```python
from build123d import *

# Parameters (mm, degrees)
SKETCH1_W                       = 123.5
SKETCH1_H                       = 220
BLOCO_DEPTH                     = 20.4
SKETCH2_R                       = 17.5
FURO_35_PASSANTE_DEPTH          = 254.117383836
SKETCH2_4_R                     = 30
SKETCH2_4_R_2                   = 17.5
REBAIXO_60X10_DEPTH             = 10
REBAIXO_M6_PASSANTE_D           = 6.6
REBAIXO_M6_PASSANTE_CBORE_D     = 11
REBAIXO_M6_PASSANTE_CBORE_DEPTH = 6
FURO_M5X0_8_PASSANTE_D          = 4.2


with BuildPart() as part:
    # Sketch1 → Bloco (new body)
    with BuildSketch(Plane(origin=(0, 0, 0), x_dir=(1, 0, 0), z_dir=(0, 1, 0))):
        with Locations((61.75, 110)):
            Rectangle(SKETCH1_W, SKETCH1_H)
    extrude(amount=-BLOCO_DEPTH)

    # Sketch2 → Furo _35 Passante (cut, through all)
    with BuildSketch(Plane(origin=(0, -20.4, 0), x_dir=(-1, 0, 0), z_dir=(0, -1, 0))):
        with Locations(Location((-23.5, 110, 0), (0, 0, 90))):
            Circle(SKETCH2_R)
    extrude(amount=-FURO_35_PASSANTE_DEPTH, mode=Mode.SUBTRACT)

    # Sketch2_4 → Rebaixo _60x10 (cut)
    with BuildSketch(Plane(origin=(0, -20.4, 0), x_dir=(-1, 0, 0), z_dir=(0, -1, 0))):
        with Locations((-23.5, 110)):
            Circle(SKETCH2_4_R)
        with Locations(Location((-23.5, 110, 0), (0, 0, 90))):
            Circle(SKETCH2_4_R_2, mode=Mode.SUBTRACT)
    extrude(amount=-REBAIXO_60X10_DEPTH, mode=Mode.SUBTRACT)

    # Rebaixo M6 - Passante (through all)
    with Locations(Plane(origin=(0, 0, 0), x_dir=(1, 0, 0), z_dir=(0, 1, 0))):
        with Locations((117.25, 10), (117.25, 110), (117.25, 210)):
            CounterBoreHole(REBAIXO_M6_PASSANTE_D / 2, REBAIXO_M6_PASSANTE_CBORE_D / 2, REBAIXO_M6_PASSANTE_CBORE_DEPTH)

    # Furo M5x0.8 - Passante (through all)
    with Locations(Plane(origin=(0, 0, 0), x_dir=(1, 0, 0), z_dir=(0, 1, 0))):
        with Locations((53.75, 10), (117.25, 50), (117.25, 170), (53.75, 210)):
            Hole(FURO_M5X0_8_PASSANTE_D / 2)


solid = part.part
```
For this review, take the finished solid that the model builds, in its own axes (mm). A direction names the side the tool comes from. Round coordinates to 2 decimals unless told otherwise and drop trailing zeros. Loops run counter-clockwise (first coordinate to the right, second up) from the corner with the lowest first, then second, coordinate; pieces in that order, holes last.
Q1. To check wall thickness, follow line 1 along Z through (x, y) = (117.25, -15.5); line 2 along Z through (x, y) = (117.25, -2.2); line 3 along X through (y, z) = (-7.25, -110). State the ranges of each line that lie inside material, in increasing order.
Result sheet:
line 1: z = -220 to -213.3, -206.7 to -172.1, -167.9 to -113.3, -106.7 to -52.1, -47.9 to -13.3, -6.7 to 0
line 2: z = -220 to -215.5, -204.5 to -172.1, -167.9 to -115.5, -104.5 to -52.1, -47.9 to -15.5, -4.5 to 0
line 3: x = 0 to 6, 41 to 113.95, 120.55 to 123.5
Q2. Add section C-C on x = 36. Write out the cut boundary in (y, z), plus the area to 3 significant figures.
Result sheet:
outline: (-20.4, -220) - (0, -220) - (0, -122.25) - (-10.4, -122.25) - (-10.4, -137.27) - (-20.4, -137.27) - close; (-20.4, -82.73) - (-10.4, -82.73) - (-10.4, -97.75) - (0, -97.75) - (0, 0) - (-20.4, 0) - close
area: 3,690 mm2
Q3. Add section B-B on z = -50. Write out the cut boundary in (x, y), plus the area to 3 significant figures.
Result sheet:
outline: (0, -20.4) - (115.15, -20.4) - (115.15, 0) - (0, 0) - close; (119.35, -20.4) - (123.5, -20.4) - (123.5, 0) - (119.35, 0) - close
area: 2,430 mm2
Q4. Insertion check: pin 1 Ø5.5 at (x, z) = (117.5, -107.5) entering from +Y. The pin has a flat end and moves straight along its axis. Give the tip position at first contact, or say it passes through.
Result sheet:
pin 1: stops at y = -6
Q5. Add section A-A on z = -110. Write out the cut boundary in (x, y), plus the area to 3 significant figures.
Result sheet:
outline: (0, -10.4) - (6, -10.4) - (6, 0) - (0, 0) - close; (41, -10.4) - (53.5, -10.4) - (53.5, -20.4) - (113.95, -20.4) - (113.95, -6) - (111.75, -6) - (111.75, 0) - (41, 0) - close; (120.55, -20.4) - (123.5, -20.4) - (123.5, 0) - (122.75, 0) - (122.75, -6) - (120.55, -6) - close
area: 1,460 mm2
Q6. Mouldability with a two-part tool opening along X and no side actions: class faces 4 (the face through (120.547, -13.301, -10.145)), 5 (the face through (123.5, -10, -108)), 6 (the face through (61, -20.4, -112)) as +X half, -X half, draft (parallel to the pull), parting line (faces both ways), or undercut.
Result sheet:
face 4: undercut
face 5: +X half
face 6: draft
Q7. Add section D-D on y = -16. Write out the cut boundary in (x, z), plus the area to 4 significant figures.
Result sheet:
outline: (0, -220) - (123.5, -220) - (123.5, 0) - (0, 0) - (0, -91.35) arc R30 cw (long way) to (0, -128.65) - close; hole circle Ø4.2 at (53.75, -210); hole circle Ø4.2 at (53.75, -10); hole circle Ø6.6 at (117.25, -210); hole circle Ø6.6 at (117.25, -110); hole circle Ø6.6 at (117.25, -10); hole circle Ø4.2 at (117.25, -170); hole circle Ø4.2 at (117.25, -50)
area: 24,350 mm2
Q8. Machinability: for faces 1 (the face through (61, -10, -220)), 2 (the face through (53.48, -15.47, -111.04)), 3 (the face through (117, -6, -6)), which of the approach directions +Z, -Z, +X, -X, +Y, -Y give a long, thin tool a straight path to every point of the face, cutting with its end or side? Answer none if there is none.
Result sheet:
face 1: -Z, +X, -X, +Y, -Y
face 2: -Y
face 3: +Y
